Study the drawing (mm; zero at the part's minimum x, y, z) and answer. A direction names the side the tool comes from. Coordinates: 2 decimals unless noted, no trailing zeros. Order: outer loops, then holes, each group sorted by start corner. A loop starts at its lowest first (then second) coordinate and runs counter-clockwise, first axis right, second up. Notation, with made-up numbers: M 77.25,82 L 121.25,82 A21 ccw 121.25,87 Z; hole C 85.5,-19.5 d5. An arc over 180 degrees is marked long. Use a Markdown table: item, result. Add a question column.
1) Find the intervals of material crossed by probe 1 along X at (y, z) = (7.5, 125); probe 2 along Z at (x, y) = (131, 7.25); probe 3 along X at (y, z) = (17.25, 56.5), in increasing order. Write a range as [from, to].
2) Find section C-C on y = 3.5. Write down the section's boundary in (x, z).
3) Find section A-A on x = 70. Write down the section's boundary in (y, z).
4) For the marked faces 1 and 2, determine the directions among +Z, -Z, +X, -X, +Y, -Y from which every point of the face is accessible in a straight line to the end or side of a thin tool.
5) Find section B-B on z = 50. Write down the section's boundary in (x, y).
6) Each of these flat-tipped pins is pushed along its axis until it touches: pin 1 Ø1.2 at (x, z) = (131, 15) entering from -Y; pin 2 Ø2.5 at (x, z) = (9, 125) entering from +Y. Where does it stop, or does it pass through?
7) The mould has two halves that part along Z. Classify the marked faces 3, 4 and 5: released by +Z, released by -Z, zero draft, split by the parting line, or undercut.
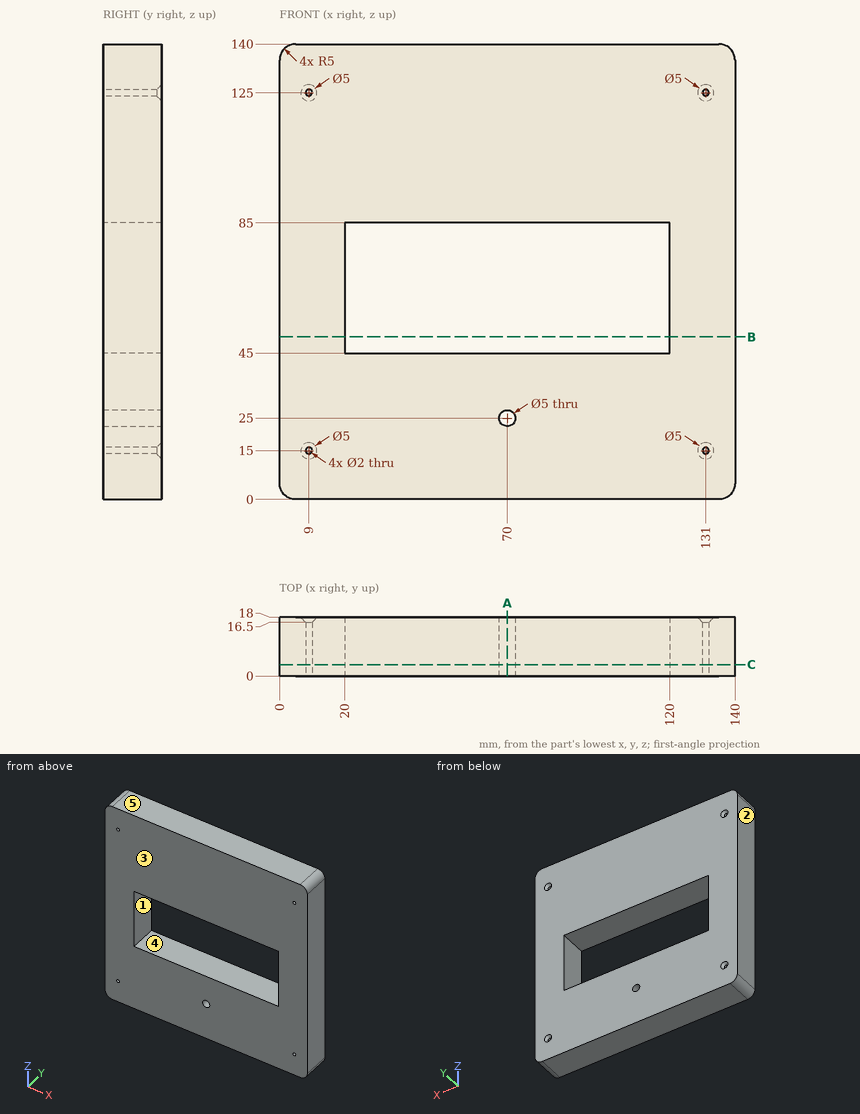
Check result:
| question | item | result |
|---|---|---|
| 1 | probe 1 | x = [0, 8], [10, 130], [132, 140] |
| 1 | probe 2 | z = [0, 14], [16, 124], [126, 140] |
| 1 | probe 3 | x = [0, 20], [120, 140] |
| 2 | outline | M 0,5 A5 ccw 5,0 L 135,0 A5 ccw 140,5 L 140,135 A5 ccw 135,140 L 5,140 A5 ccw 0,135 Z; hole C 9,15 d2; hole C 9,125 d2; hole M 20,45 L 120,45 L 120,85 L 20,85 Z; hole C 70,25 d5; hole C 131,15 d2; hole C 131,125 d2 |
| 3 | outline | M 0,0 L 18,0 L 18,22.5 L 0,22.5 Z; M 0,27.5 L 18,27.5 L 18,45 L 0,45 Z; M 0,85 L 18,85 L 18,140 L 0,140 Z |
| 4 | face 1 | +Y, -Y |
| 4 | face 2 | +Z, -Z, -X, +Y, -Y |
| 5 | outline | M 0,0 L 20,0 L 20,18 L 0,18 Z; M 120,0 L 140,0 L 140,18 L 120,18 Z |
| 6 | pin 1 | passes through |
| 6 | pin 2 | stops at y = 16.75 |
| 7 | face 3 | zero draft |
| 7 | face 4 | undercut |
| 7 | face 5 | released by +Z |
